Autodesk Inventor part; units mm, degrees
ref_plane "Start plane" through (0, 0, 0.16) normal (0, 0, 1) x (1, 0, 0)
ref_plane "End plane" through (0, 0, 499.84) normal (0, 0, 1) x (1, 0, 0)
ref_plane "Work Plane11" through (-6, 4, 0.16) normal (0.7071, 0, -0.7071) x (-0.7071, 0, -0.7071)
ref_plane "Start plane" through (0, 0, 0.16) normal (0, 0, 1) x (1, 0, 0)
ref_plane "End plane" through (0, 0, 499.84) normal (0, 0, 1) x (1, 0, 0)
sketch "Sketch" plane through (0, 0, 0) normal (0, 0, 1) x (1, 0, 0)
  line L0 (-3, 0.5) -> (-3, 12)
  line L1 (-6, 14) -> (-5, 14)
  line L2 (-6, -6) -> (-6, 14)
  line L3 (-6, -6) -> (14, -6)
  line L4 (14, -5) -> (14, -6)
  line L5 (0.5, -3) -> (12, -3)
  arc A0 (-3, 0.5) -> (0.5, -3) centre (0.5, 0.5) ccw
  arc A1 (-3, 12) -> (-5, 14) centre (-5, 12) ccw
  arc A2 (14, -5) -> (12, -3) centre (12, -5) ccw
  line L6 (0, 18.4971) -> (0, -10.0828) construction
  line L7 (-10.0828, 0) -> (18.4971, 0) construction
  point P0 (-3, -3)
  point P1 (-3, 14)
  point P2 (14, -3)
  dimension "d4" = 20
  dimension "d6" = 20
  dimension "d8" = 3
  dimension "d10" = 3
  dimension "d17" = 3.5
  dimension "d18" = 2
  dimension "d19" = 6
  dimension "d20" = 6
extrude "Body" add sketch "Sketch" along normal up to surface (499.68 mm away) from surface at 0.16
sketch "Sketch3" plane through (0, 0, 0) normal (0, 0, 1) x (1, 0, 0)
  line L0 (0, 0) -> (10, 0)
ref_plane "Work Plane10" through (0, 0, 0) normal (0, -1, 0) x (1, 0, 0)
sketch "Sketch4" plane through (0, 0, 0) normal (0, -1, 0) x (1, 0, 0)
  line L0 (-2, 0.16) -> (12, 0.16)
  line L1 (-2, 499.84) -> (12, 499.84)
  dimension "d24" = 499.68
ref_plane "Work Plane11" through (-6, 4, 0.16) normal (0.7071, 0, -0.7071) x (-0.7071, 0, -0.7071)
split "Split1" plane through (-6, 4, 0.16) removes the side toward (0.7071, 0, -0.7071)
ref_plane "Work Plane12" through (-6, 4, 499.84) normal (0.7071, 0, 0.7071) x (0.7071, 0, -0.7071)
split "Split2" plane through (-6, 4, 499.84) removes the side toward (0.7071, 0, 0.7071)
equation "\"d4\" = b"
equation "\"d6\" = b"
equation "\"d17\" = R"
equation "\"d18\" = R1"
equation "\"d19\" = ex"
equation "\"d20\" = d19"
equation "\"d11\" = G_L"
equation "\"b\" = 20"
equation "\"ParT\" = 3"
equation "\"R\" = 3.5"
equation "\"R1\" = 2"
equation "\"G_L\" = d24"
equation "\"ex\" = 6"
equation "\"G_OFFSET_START\" = -0.16"
equation "\"G_OFFSET_END\" = -0.16"
equation "\"d21\" = -G_OFFSET_START"
equation "\"d22\" = G_OFFSET_END + B_L"
properties part number "ISO 657-1 - L20x20x3-499.68" material "Stainless Steel"
Work out the finished part from the listing and answer in its coordinate system (mm). A direction names the side the tool comes from. Give positions to 0.01 mm unless a question says otherwise; leave off trailing zeros. Order: outer loops, then holes, each group sorted by start corner. A loop starts at its lowest first (then second) coordinate and runs counter-clockwise, first axis right, second up. Notation, with made-up numbers: (-7.5, 30) -> (51.5, 30) arc R26 ccw to (51.5, 62) -> close; hole circle Ø2 at (27.5, 84.5). An arc over 180 degrees is marked (long way). Answer as a JSON object with one key per item and string values. Group by question number.
1. Section A-A on z = 364 is taken. Determine the outline of the cut face in (x, y), plus the area to 3 significant figures.
2. Section B-B on y = 8.5 is taken. Determine the outline of the cut face in (x, z).
3. Section C-C on x = 6.25 is taken. Determine the outline of the cut face in (y, z), plus the area to 3 significant figures.
4. Consider line 1 along Y through (x, z) = (11.25, 23); line 2 along Z through (x, y) = (-5, 4.75). Determine where each line is inside the solid, lowest interval first. Write a range as [from, to].
5. Flat-ended cylindrical pins translate along their axes: pin 1 Ø6 at (y, z) = (4, 132.5) entering from +X; pin 2 Ø4 at (x, y) = (-0.5, 2) entering from -Z; pin 3 Ø12 at (x, y) = (0.5, -3) entering from -Z. Find the tip coordinate at first contact, or state that the pin passes through.
6. A tool of negligible diameter and unlimited length cuts with its end or side. For faces 1 (the flat face through (4, -6, 247)), 2 (the flat face through (-3, 6, 247)), from which of +Z, -Z, +X, -X, +Y, -Y can it reach the whole face along a straight path? Write none if from no direction.
Result sheet:
{
 "1": {"outline": "(-6, -6) -> (14, -6) -> (14, -5) arc R2 ccw to (12, -3) -> (0.5, -3) arc R3.5 cw to (-3, 0.5) -> (-3, 12) arc R2 ccw to (-5, 14) -> (-6, 14) -> close", "area": "112 mm^2"},
 "2": {"outline": "(-6, 0.16) -> (-3, 3.16) -> (-3, 496.84) -> (-6, 499.84) -> close"},
 "3": {"outline": "(-6, 12.41) -> (-3, 12.41) -> (-3, 487.59) -> (-6, 487.59) -> close", "area": "1,430 mm^2"},
 "4": {"line 1": "y = [-6, -3]", "line 2": "z = [1.16, 498.84]"},
 "5": {"pin 1": "stops at x = -3", "pin 2": "passes through", "pin 3": "stops at z = 0.66"},
 "6": {"face 1": "+Z, -Z, +X, -X, -Y", "face 2": "+Z, -Z, +X, +Y"}
}
